Check sheet for the drawn part. Datum: minimum x, y, z corner. Units: mm. A direction names the side the tool comes from. Coordinates: 2 decimals unless noted, no trailing zeros. Order: outer loops, then holes, each group sorted by start corner. A loop starts at its lowest first (then second) coordinate and runs counter-clockwise, first axis right, second up. Notation, with made-up numbers: (47.25, 30.5) -> (75.25, 30.5) arc R32 ccw to (75.25, 60.5) -> close; hole circle Ø1 at (-16.5, -1.75). An arc over 180 degrees is marked (long way). Answer as CSV lines item,"result".
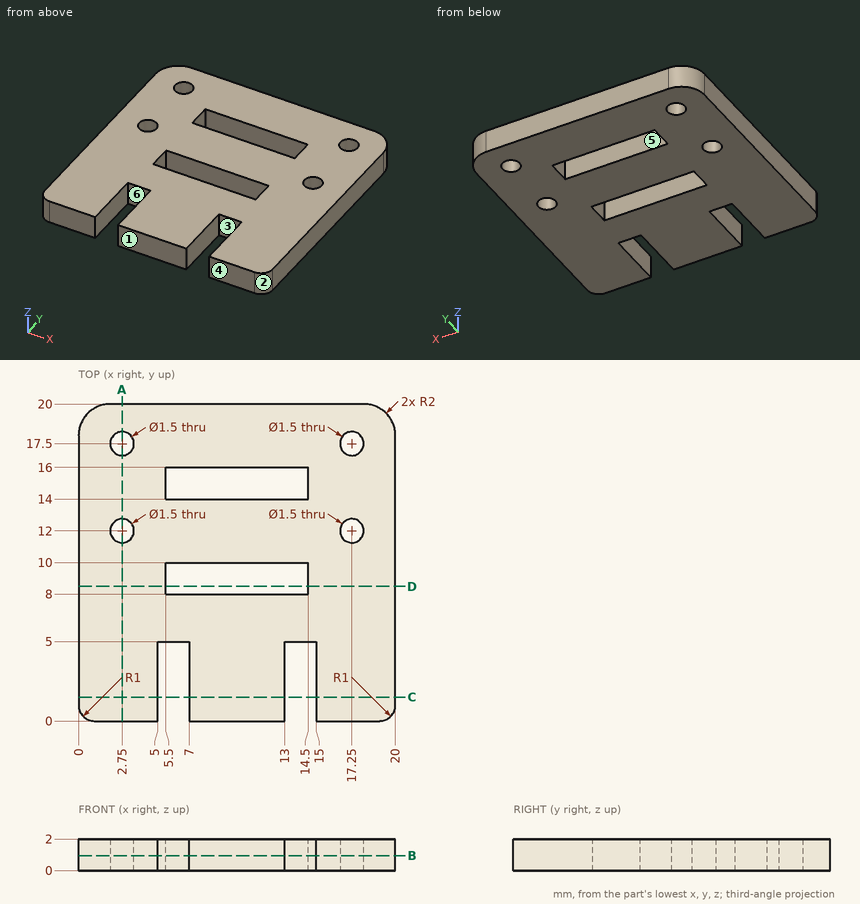
Item 1: Section check D-D, the plane y = 8.5. Record the boundary of the cut face in (x, z).
Answer list:
outline,"(0, 0) -> (5.5, 0) -> (5.5, 2) -> (0, 2) -> close; (14.5, 0) -> (20, 0) -> (20, 2) -> (14.5, 2) -> close"
Item 2: Thickness scan on line 1 (Y direction, x = 7.25, z = 0.2); line 2 (X direction, y = 4.75, z = 1.5); line 3 (Y direction, x = 17.25, z = 0.5). Record the ranges inside material, lowest first.
Answer list:
line 1,"0 to 8, 10 to 14, 16 to 20"
line 2,"0 to 5, 7 to 13, 15 to 20"
line 3,"0 to 11.25, 12.75 to 16.75, 18.25 to 20"
Item 3: Section check A-A, the plane x = 2.75. Record the boundary of the cut face in (y, z), plus the area to 3 significant figures.
Answer list:
outline,"(0, 0) -> (11.25, 0) -> (11.25, 2) -> (0, 2) -> close; (12.75, 0) -> (16.75, 0) -> (16.75, 2) -> (12.75, 2) -> close; (18.25, 0) -> (20, 0) -> (20, 2) -> (18.25, 2) -> close"
area,"34.0 mm2"
Item 4: Section check C-C, the plane y = 1.5. Record the boundary of the cut face in (x, z), plus the area to 3 significant figures.
Answer list:
outline,"(0, 0) -> (5, 0) -> (5, 2) -> (0, 2) -> close; (7, 0) -> (13, 0) -> (13, 2) -> (7, 2) -> close; (15, 0) -> (20, 0) -> (20, 2) -> (15, 2) -> close"
area,"32.0 mm2"
Item 5: Release check for a two-part mould opening along X. For the marked faces 1, 2 and 3 record: +X half, -X half, draft (parallel to the pull), parting line (faces both ways), or undercut.
Answer list:
face 1,"draft"
face 2,"+X half"
face 3,"undercut"
Item 6: Section check B-B, the plane z = 0.95. Record the boundary of the cut face in (x, y).
Answer list:
outline,"(0, 1) arc R1 ccw to (1, 0) -> (5, 0) -> (5, 5) -> (7, 5) -> (7, 0) -> (13, 0) -> (13, 5) -> (15, 5) -> (15, 0) -> (19, 0) arc R1 ccw to (20, 1) -> (20, 18) arc R2 ccw to (18, 20) -> (2, 20) arc R2 ccw to (0, 18) -> close; hole circle Ø1.5 at (2.75, 12); hole circle Ø1.5 at (2.75, 17.5); hole (5.5, 8) -> (14.5, 8) -> (14.5, 10) -> (5.5, 10) -> close; hole (5.5, 14) -> (14.5, 14) -> (14.5, 16) -> (5.5, 16) -> close; hole circle Ø1.5 at (17.25, 12); hole circle Ø1.5 at (17.25, 17.5)"
Item 7: Tool access check on the marked faces 4, 5 and 6. Record the directions out of +Z, -Z, +X, -X, +Y, -Y that give a thin tool (end or side, any length) a straight path to the whole face; none if there is none.
Answer list:
face 4,"+Z, -Z, +X, -X, -Y"
face 5,"+Z, -Z"
face 6,"+Z, -Z, -Y"
Item 8: Depth check by flat-ended pin: pin 1 Ø1 at (x, z) = (8.5, 1) entering from -Y; pin 2 Ø1 at (x, z) = (6, 1) entering from -Y. Enter the tip coordinate at first touch or a pass-through.
Answer list:
pin 1,"y = 0"
pin 2,"y = 5"
